Design review of the part shown in the three views and the two pictorial views. Dimensions are in mm from the part's minimum x, y and z. Round coordinates to 2 decimals unless told otherwise and drop trailing zeros. Write each loop counter-clockwise with the first axis right and the second up, starting at its lowest first coordinate (ties: lowest second). Pieces come first, ordered by that corner, then holes. Notation, with made-up numbers: (89, -40) - (102, -40) arc R17 ccw to (102, -27) - close; hole circle Ø4 at (49, 47.25). An arc over 180 degrees is marked (long way). Use one line per item in the form item = value.
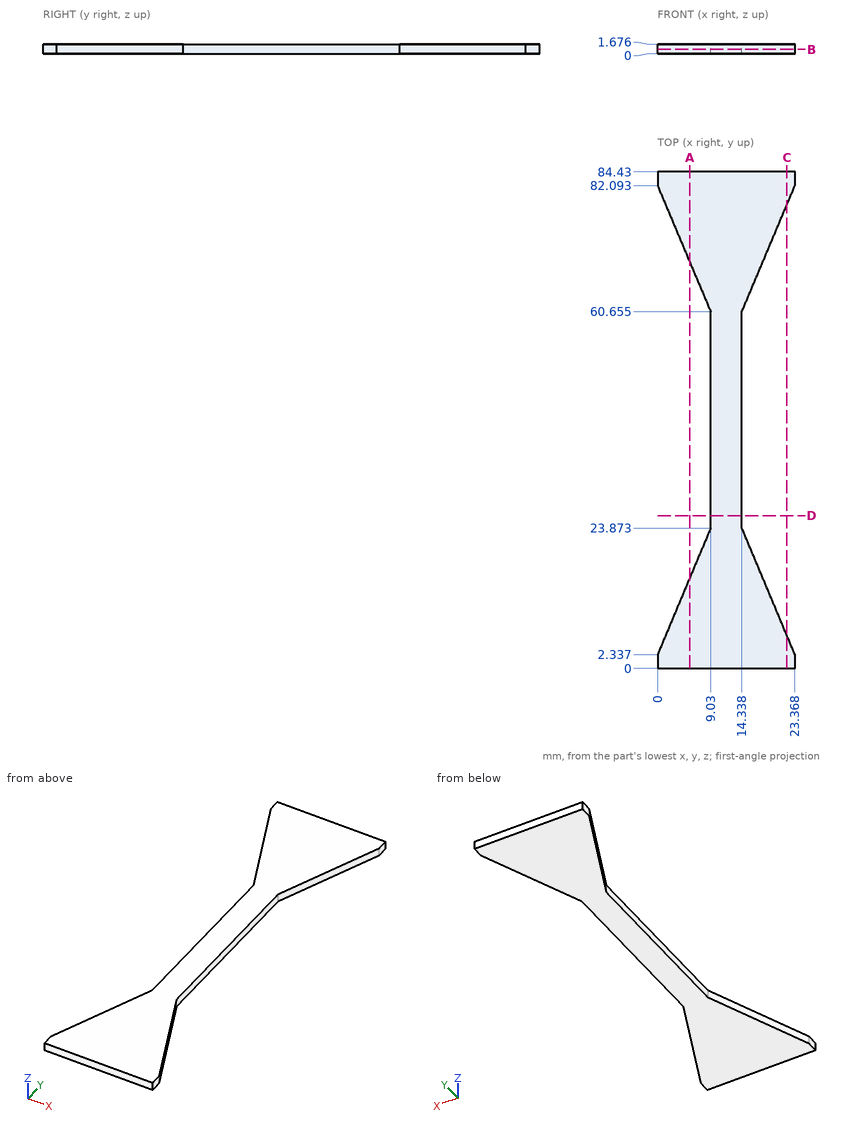
Q1. We need section D-D on y = 26. Write out the cut boundary in (x, z).
Calculated:
outline = (9.03, 0) - (14.34, 0) - (14.34, 1.68) - (9.03, 1.68) - close
Q2. To check wall thickness, follow line 1 along X through (y, z) = (32, 0.4); line 2 along Y through (x, z) = (6.75, 1.55) (1 decimal); line 3 along Y through (x, z) = (17.25, 0.6) (1 decimal). State the ranges of each line that lie inside material, in increasing order. Write a range as from..to.
Calculated:
line_1 = 9.03..14.34
line_2 = 0..18.4, 66.1..84.4
line_3 = 0..16.9, 67.6..84.4
Q3. We need section C-C on x = 22. Write out the cut boundary in (y, z) (1 decimal).
Calculated:
outline = (0, 0) - (5.6, 0) - (5.6, 1.7) - (0, 1.7) - close; (78.8, 0) - (84.4, 0) - (84.4, 1.7) - (78.8, 1.7) - close
Q4. We need section B-B on z = 0.75. Write out the cut boundary in (x, y) (1 decimal).
Calculated:
outline = (0, 0) - (23.4, 0) - (23.4, 2.3) - (14.3, 23.9) - (14.3, 60.7) - (23.4, 82.1) - (23.4, 84.4) - (0, 84.4) - (0, 82.1) - (9, 60.7) - (9, 23.9) - (0, 2.3) - close
Q5. For P1, Ø1, axis at y = 23.5, z = 1, coming from the +X side (1 decimal), flat-tipped, find the tip position at first contact; note if it passes through.
Calculated:
P1 = 14.7
Q6. We need section A-A on x = 5.5. Write out the cut boundary in (y, z) (1 decimal).
Calculated:
outline = (0, 0) - (15.5, 0) - (15.5, 1.7) - (0, 1.7) - close; (69, 0) - (84.4, 0) - (84.4, 1.7) - (69, 1.7) - close
